Part model, mm, in its own coordinate system. Face numbers are marked on the shaded views. Give positions to 0.01 mm unless a question says otherwise; leave off trailing zeros. Write each loop counter-clockwise with the first axis right and the second up, starting at its lowest first coordinate (ties: lowest second). Pieces come first, ordered by that corner, then holes.
Solid Edge part; units mm, degrees
sketch "Sketch1" plane through (0, 0, 0) normal (0, 0, 1) x (1, 0, 0)
  circle A0 centre (0, 0) radius 2
  line L0 (-4, 0) -> (-4, 4)
  line L1 (-4, 4) -> (4, 4)
  line L2 (4, 4) -> (4, 0)
  arc A1 (4, 0) -> (-4, 0) centre (0, 0) cw
extrude "Protrusion1" add sketch "Sketch1" along normal blind 6
sketch "Sketch2" plane through (0, 0, 6) normal (0, 0, 1) x (1, 0, 0)
  line L0 (-4, 3) -> (4, 3)
  line L1 (4, 3) -> (4, 4)
  line L2 (4, 4) -> (-4, 4)
  line L3 (-4, 4) -> (-4, 3)
  dimension "D1" = 4
extrude "Extrusionsausschnitt_1" cut sketch "Sketch2" against normal blind 1
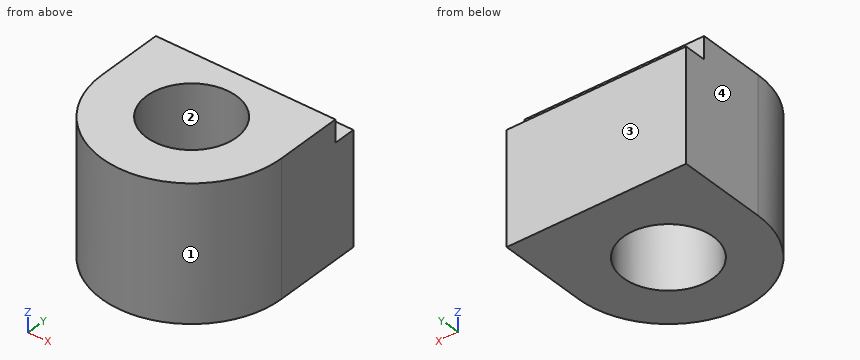
1) Saw through at C-C (y = 1.5). Write the cut outline in (x, z).
Check result:
outline: (-4, 0) - (-1.32, 0) - (-1.32, 6) - (-4, 6) - close; (1.32, 0) - (4, 0) - (4, 6) - (1.32, 6) - close
2) Saw through at D-D (x = 1.25). Write the cut outline in (y, z), and give its area (3 significant figures).
Check result:
outline: (-3.8, 0) - (-1.56, 0) - (-1.56, 6) - (-3.8, 6) - close; (1.56, 0) - (4, 0) - (4, 5) - (3, 5) - (3, 6) - (1.56, 6) - close
area: 27.1 mm2
3) Saw through at B-B (z = 4.1). Write the cut outline in (x, y), and give its area (3 significant figures).
Check result:
outline: (-4, 0) arc R4 ccw to (4, 0) - (4, 4) - (-4, 4) - close; hole circle Ø4 at (0, 0)
area: 44.6 mm2
4) Mould opens along Y. For the marked faces 1, 2, 3 and 4 say: +Y half, -Y half, draft (parallel to the pull), parting line (faces both ways), or undercut.
Check result:
face 1: -Y half
face 2: undercut
face 3: +Y half
face 4: draft
5) Flat gauge pins, fed straight in: P1, Ø4.5, axis at x = 0, y = 0, coming from the +Z side; P2, Ø0.8, axis at x = -1.5, y = 3.5, coming from the +Z side; P3, Ø2, axis at y = -1.5, z = 1.5, coming from the -X side. Where does each tip first touch, or does it go through?
Check result:
P1: stops at z = 6
P2: stops at z = 5
P3: stops at x = -3.97
6) Saw through at A-A (x = 0). Write the cut outline in (y, z), and give its area (3 significant figures).
Check result:
outline: (-4, 0) - (-2, 0) - (-2, 6) - (-4, 6) - close; (2, 0) - (4, 0) - (4, 5) - (3, 5) - (3, 6) - (2, 6) - close
area: 23.0 mm2
7) Drill centre lines: L1, parallel to Y at x = 0, z = 4.3; L2, parallel to X at y = -1.75, z = 2.45; L3, parallel to X at y = 1.75, z = 3.4. Where is each one in solid material? Low to high.
Check result:
L1: y = -4 to -2, 2 to 4
L2: x = -3.6 to -0.97, 0.97 to 3.6
L3: x = -4 to -0.97, 0.97 to 4
